```python
from build123d import *

# Parameters (mm, degrees)
BOSS_EXTRUDE1_DEPTH = 4.8
FILLET1_R           = 2
SKETCH2_R           = 1.5
SKETCH2_R_2         = 1.614746674
CUT_EXTRUDE1_DEPTH  = 10


with BuildPart() as part:
    # Sketch1 → Boss-Extrude1 (new body)
    with BuildSketch(Plane(origin=(0, 0, 0), x_dir=(1, 0, 0), z_dir=(0, 1, 0))):
        with BuildLine():
            Line((-7.626177736, 16.493998363), (-8.85052129, 21.762554574))
            Line((-8.85052129, 21.762554574), (-2.268963588, 40.648610229))
            Line((-2.268963588, 40.648610229), (2.386475485, 43.745687988))
            ThreePointArc((2.386475485, 43.745687988), (9.13418612, 45.073723969), (12.966474819, 50.784139165))
            Line((12.966474819, 50.784139165), (17.54572209, 53.830529559))
            Line((17.54572209, 53.830529559), (24.824248009, 52.021369411))
            ThreePointArc((24.824248009, 52.021369411), (27.493630804, 49.405257048), (30.937059303, 47.951830552))
            ThreePointArc((30.937059303, 47.951830552), (33.863857438, 48.029479081), (36.594025871, 49.08700305))
            Line((36.594025871, 49.08700305), (43.386576908, 47.395479947))
            Line((43.386576908, 47.395479947), (44.534165754, 46.483148945))
            ThreePointArc((44.534165754, 46.483148945), (45.928151501, 43.341073181), (48.215256064, 40.774949823))
            ThreePointArc((48.215256064, 40.774949823), (51.212544898, 39.439353475), (54.434824491, 38.819295269))
            Line((54.434824491, 38.819295269), (56.78893552, 36.959682067))
            Line((56.78893552, 36.959682067), (56.78893552, 22.3328147))
            Line((56.78893552, 22.3328147), (48, 0))
            Line((48, 0), (0, 0))
            Line((0, 0), (-3.788950591, 6.040862349))
            ThreePointArc((-3.788950591, 6.040862349), (-4.118018176, 11.850934579), (-7.626177736, 16.493998363))
        make_face()
        with BuildLine():
            Line((5.26881179, 9.725992339), (41.26881179, 9.725992339))
            Line((41.26881179, 9.725992339), (46.78893552, 23.7527081))
            Line((46.78893552, 23.7527081), (46.78893552, 31.7527081))
            ThreePointArc((46.78893552, 31.7527081), (41.625067619, 33.731492126), (38.544083054, 38.323730364))
            ThreePointArc((38.544083054, 38.323730364), (29.126849272, 38.096934575), (20.817558646, 42.534435867))
            ThreePointArc((20.817558646, 42.534435867), (14.72472781, 36.782412637), (6.864667897, 33.879342365))
            Line((6.864667897, 33.879342365), (2.751194333, 22.075557581))
            Line((2.751194333, 22.075557581), (2.085687611, 19.952561058))
            ThreePointArc((2.085687611, 19.952561058), (5.175485312, 15.305617866), (5.26881179, 9.725992339))
        make_face(mode=Mode.SUBTRACT)
    extrude(amount=BOSS_EXTRUDE1_DEPTH)

    # Fillet1
    fillet1_edges = [part.edges().sort_by_distance(p)[0] for p in [
        (48, 2.4, 0),
        (0, 2.4, 0),
    ]]
    fillet(fillet1_edges, radius=FILLET1_R)

    # Sketch2 → Cut-Extrude1 (cut)
    with BuildSketch(Plane(origin=(0, 4.8, 0), x_dir=(1, 0, 0), z_dir=(0, 1, 0))):
        with Locations((27.493630804, 45.905257048)):
            Circle(SKETCH2_R)
        with Locations((2.124845143, 5.7)):
            Circle(SKETCH2_R_2)
        with Locations((37.26881179, 4.8)):
            Circle(SKETCH2_R)
    extrude(amount=-CUT_EXTRUDE1_DEPTH, mode=Mode.SUBTRACT)


solid = part.part
```
Geometry: final body of the model. Coordinates: model frame, mm. A direction names the side the tool comes from. Round coordinates to 2 decimals unless told otherwise and drop trailing zeros. Order: outer loops, then holes, each group sorted by start corner. A loop starts at its lowest first (then second) coordinate and runs counter-clockwise, first axis right, second up. Notation, with made-up numbers: M 5.25,-37 L 56.25,-37 A31 ccw 56.25,-5 Z; hole C 3,-2.75 d1. An arc over 180 degrees is marked long. Use one line per item in the form item = value. Start each with the question number.
Q1. Access query for faces 1 (the face through (-4.1, 2.4, -11.8)), 2 (the face through (2.423, 2.366, -21.029)), 3 (the face through (27.45, 2.366, -49.435)). Directions: +Z, -Z, +X, -X, +Y, -Y. A direction counts if a zero-diameter tool reaches every point of the face in a straight line with its end or side. Return the directions, or none.
Q2. Mould query, pull axis Z, two halves, no side actions, for faces 4 (the face through (41.69, 2.37, -33.68)), 5 (the face through (56.789, 2, -30)), 6 (the face through (51.169, 2.366, -39.453)). Classes: +Z half, -Z half, draft (parallel to the pull), parting line (faces both ways), or undercut.
Q3. Cut plane C-C (x = 45.5). Return loops of the section in (y, z), and give its area (3 significant figures).
Q4. Pin query (flat end, axial travel): pin 1 Ø2.5 at (x, y) = (25.5, 2.5) entering from -Z; pin 2 Ø2.5 at (y, z) = (1.5, -27) entering from -X. Return the tip coordinate at first contact, or that it passes through.
Q5. Cut plane D-D (z = -27.5). Return loops of the section in (x, y), and give its area (3 significant figures).
Q6. Cut plane A-A (z = -4.8). Return loops of the section in (x, y), and give its area (3 significant figures).
Q7. Cut plane B-B (y = 1.75). Count the separate pieces of the cut face and the enclosed holes in it, and give its area (3 significant figures).
Q8. Material intervals for line 1 (Z direction, x = 28.5, y = 3.4); line 2 (X direction, y = 1.55, z = -5.7); line 3 (X direction, y = 3.55, z = -24.5), sorted ascending. Write a range as [from, to].
Geometry results:
q1.face_1 = -X, +Y, -Y
q1.face_2 = +Y, -Y
q1.face_3 = -Z, +Y, -Y
q2.face_4 = undercut
q2.face_5 = draft
q2.face_6 = -Z half
q3.outline = M 0,-44.06 L 4.8,-44.06 L 4.8,-31.92 L 0,-31.92 Z; M 0,-20.48 L 4.8,-20.48 L 4.8,0 L 0,0 Z
q3.area = 157 mm^2
q4.pin_1 = -52.16
q4.pin_2 = -7.46
q5.outline = M -6.85,0 L 4.64,0 L 4.64,4.8 L -6.85,4.8 Z; M 46.79,0 L 56.79,0 L 56.79,4.8 L 46.79,4.8 Z
q5.area = 103 mm^2
q6.outline = M -3.01,0 L 0.78,0 L 0.78,4.8 L -3.01,4.8 Z; M 3.47,0 L 35.77,0 L 35.77,4.8 L 3.47,4.8 Z; M 38.77,0 L 49.89,0 L 49.89,4.8 L 38.77,4.8 Z
q6.area = 227 mm^2
q7.separate_pieces = 1
q7.enclosed_holes = 4
q7.area = 1,630 mm^2
q8.line_1 = [-48.82, -47.02], [-44.79, -38.26], [-9.73, 0]
q8.line_2 = [-3.58, 0.51], [3.74, 36.07], [38.47, 50.24]
q8.line_3 = [-7.9, 3.6], [46.79, 56.79]
